```python
from build123d import *

# Parameters (mm, degrees)
SKETCH1_W                                        = 50.8
SKETCH1_H                                        = 25.4
BOSS_EXTRUDE1_DEPTH                              = 25.4
CBORE_FOR_1_4_SOCKET_HEAD_CAP_SCREW1_D           = 6.7564
CBORE_FOR_1_4_SOCKET_HEAD_CAP_SCREW1_CBORE_D     = 11.1125
CBORE_FOR_1_4_SOCKET_HEAD_CAP_SCREW1_CBORE_DEPTH = 19.05
SKETCH6_W                                        = 50.8
SKETCH6_H                                        = 4.7
BOSS_EXTRUDE2_DEPTH                              = 20
CBORE_FOR_M4_SBHCS1_D                            = 4.8
CBORE_FOR_M4_SBHCS1_CBORE_D                      = 8.6
CBORE_FOR_M4_SBHCS1_CBORE_DEPTH                  = 2.2
FILLET1_R                                        = 10
SKETCH15_W                                       = 50.8
SKETCH15_H                                       = 25.4
BOSS_EXTRUDE3_DEPTH                              = 20
SKETCH16_W                                       = 51.113320751
SKETCH16_H                                       = 27.993322013
CUT_EXTRUDE2_DEPTH                               = 12.7


with BuildPart() as part:
    # Sketch1 → Boss-Extrude1 (new body)
    with BuildSketch(Plane(origin=(0, 0, 0), x_dir=(1, 0, 0), z_dir=(0, 1, 0))):
        with Locations((2.315568022, 7.890743338)):
            Rectangle(SKETCH1_W, SKETCH1_H)
    extrude(amount=BOSS_EXTRUDE1_DEPTH)

    # CBORE for 1/4 Socket Head Cap Screw1 (through all)
    with Locations(Plane(origin=(0, 25.4, 0), x_dir=(1, 0, 0), z_dir=(0, 1, 0))):
        with Locations((-10.384431978, 7.890743338), (15.015568022, 7.890743338)):
            CounterBoreHole(CBORE_FOR_1_4_SOCKET_HEAD_CAP_SCREW1_D / 2, CBORE_FOR_1_4_SOCKET_HEAD_CAP_SCREW1_CBORE_D / 2, CBORE_FOR_1_4_SOCKET_HEAD_CAP_SCREW1_CBORE_DEPTH)

    # Sketch6 → Boss-Extrude2 (add)
    with BuildSketch(Plane(origin=(0, 25.4, 0), x_dir=(1, 0, 0), z_dir=(0, 1, 0))):
        with Locations((2.315568022, 18.240743338)):
            Rectangle(SKETCH6_W, SKETCH6_H)
    extrude(amount=BOSS_EXTRUDE2_DEPTH)

    # CBORE for M4 SBHCS1 (through all)
    with Locations(Plane.XY.offset(-15.890743338)):
        with Locations((2.315568022, 35.4)):
            CounterBoreHole(CBORE_FOR_M4_SBHCS1_D / 2, CBORE_FOR_M4_SBHCS1_CBORE_D / 2, CBORE_FOR_M4_SBHCS1_CBORE_DEPTH)

    # Fillet1
    fillet1_edges = [part.edges().sort_by_distance(p)[0] for p in [
        (27.715568022, 45.4, -18.240743338),
        (-23.084431978, 45.4, -18.240743338),
        (27.715568022, 12.7, 4.809256662),
        (-23.084431978, 12.7, 4.809256662),
    ]]
    fillet(fillet1_edges, radius=FILLET1_R)

    # Sketch15 → Boss-Extrude3 (add)
    with BuildSketch(Plane(origin=(0, 0, -20.590743338), x_dir=(-1, 0, 0), z_dir=(0, 0, -1))):
        with Locations((-2.315568022, 12.7)):
            Rectangle(SKETCH15_W, SKETCH15_H)
    extrude(amount=BOSS_EXTRUDE3_DEPTH)

    # Sketch16 → Cut-Extrude2 (cut)
    with BuildSketch(Plane(origin=(0, 25.4, 0), x_dir=(1, 0, 0), z_dir=(0, 1, 0))):
        with Locations((2.472228398, 1.894082332)):
            Rectangle(SKETCH16_W, SKETCH16_H)
    extrude(amount=-CUT_EXTRUDE2_DEPTH, mode=Mode.SUBTRACT)

    # Mirror1: part across plane


with BuildPart() as part_1:
    add(part.part)
    add(part.part.mirror(Plane(origin=(0, 0, -40.590743338), x_dir=(1, 0, 0), z_dir=(0, 0, -1))))


solid = part_1.part
```
CAD build for the part. Positions are in the model's coordinates, mm. A direction names the side the tool comes from. Round coordinates to 2 decimals unless told otherwise and drop trailing zeros. Loops run counter-clockwise (first coordinate to the right, second up) from the corner with the lowest first, then second, coordinate; pieces in that order, holes last. Notation, with made-up numbers: (71.25, 76) - (111.25, 76) arc R30 ccw to (111.25, 110) - close; hole circle Ø1 at (36.5, -19). An arc over 180 degrees is marked (long way). Return JSON: item names as keys, results as strings. Group by question number.
Q1. Band-saw the part on B-B on y = 41. Give the cut face in (x, z).
Q2. Band-saw the part on D-D on z = -26. Give the cut face in (x, y).
Q3. Band-saw the part on A-A on x = 8.5. Give the cut face in (y, z), plus the area to 3 significant figures.
Q4. Two-plate mould, pull along X, no slides. Class faces 5 (the face through (24.708, 42.548, -62.908)), 6 (the face through (2, 31, -60.591)), 7 (the face through (10.92, 9.569, -11.646)), 8 (the face through (-11.94, 3.13, -76.29)): +X half, -X half, draft (parallel to the pull), parting line (faces both ways), or undercut.
Q5. Tool access for faces 1 (the face through (4.2, 33.5, -63.091)), 2 (the face through (2, 29, -15.891)), 3 (the face through (2, 12.7, -75)), 4 (the face through (14.292, 9.569, -67.782)): list every direction of +Z, -Z, +X, -X, +Y, -Y with a clear straight run to the whole face (end or side of a thin tool).
Q6. Band-saw the part on C-C on y = 7.5. Give the cut face in (x, z), plus the area to 3 significant figures.
Q7. Flat gauge pins, fed straight in: pin 1 Ø3 at (x, z) = (-10, -6.5) entering from -Y; pin 2 Ø1 at (x, y) = (-18, 37.5) entering from -Z; pin 3 Ø10 at (x, z) = (-11.5, -46) entering from -Y; pin 4 Ø5.5 at (x, z) = (13.5, -74) entering from +Y. Where does each tip first touch, or does it go through?
Q8. Drill centre lines: line 1 along X through (y, z) = (4.5, -8); line 2 along Z through (x, y) = (3, 29.5); line 3 along Z through (x, y) = (11, 12). Where is each one in solid material? Low to high. Write a range as [from, to].
Solutions:
{
 "1": {"outline": "(-21.37, -65.29) - (26, -65.29) - (26, -60.59) - (-21.37, -60.59) - close; (-21.37, -20.59) - (26, -20.59) - (26, -15.89) - (-21.37, -15.89) - close"},
 "2": {"outline": "(-23.08, 0) - (27.72, 0) - (27.72, 25.4) - (-23.08, 25.4) - close"},
 "3": {"outline": "(0, -85.99) - (12.7, -85.99) - (12.7, -65.29) - (45.4, -65.29) - (45.4, -60.59) - (25.4, -60.59) - (25.4, -20.59) - (45.4, -20.59) - (45.4, -15.89) - (12.7, -15.89) - (12.7, 4.81) - (0, 4.81) - close", "area": "1,970 mm^2"},
 "4": {"face 5": "+X half", "face 6": "draft", "face 7": "undercut", "face 8": "undercut"},
 "5": {"face 1": "-Z", "face 2": "+Z, +X, -X, +Y", "face 3": "-Z, +X, -X, +Y", "face 4": "+Y"},
 "6": {"outline": "(-23.08, -75.99) arc R10 ccw to (-13.08, -85.99) - (17.72, -85.99) arc R10 ccw to (27.72, -75.99) - (27.72, -5.19) arc R10 ccw to (17.72, 4.81) - (-13.08, 4.81) arc R10 ccw to (-23.08, -5.19) - close; hole circle Ø11.11 at (-10.38, -73.29); hole circle Ø11.11 at (-10.38, -7.89); hole circle Ø11.11 at (15.02, -73.29); hole circle Ø11.11 at (15.02, -7.89)", "area": "4,140 mm^2"},
 "7": {"pin 1": "passes through", "pin 2": "stops at z = -65.29", "pin 3": "stops at y = 0", "pin 4": "stops at y = 6.35"},
 "8": {"line 1": "x = [-23.08, -13.76], [-7.01, 11.64], [18.39, 27.72]", "line 2": "z = [-65.29, -60.59], [-20.59, -15.89]", "line 3": "z = [-85.99, -77.13], [-69.45, -11.73], [-4.05, 4.81]"}
}
